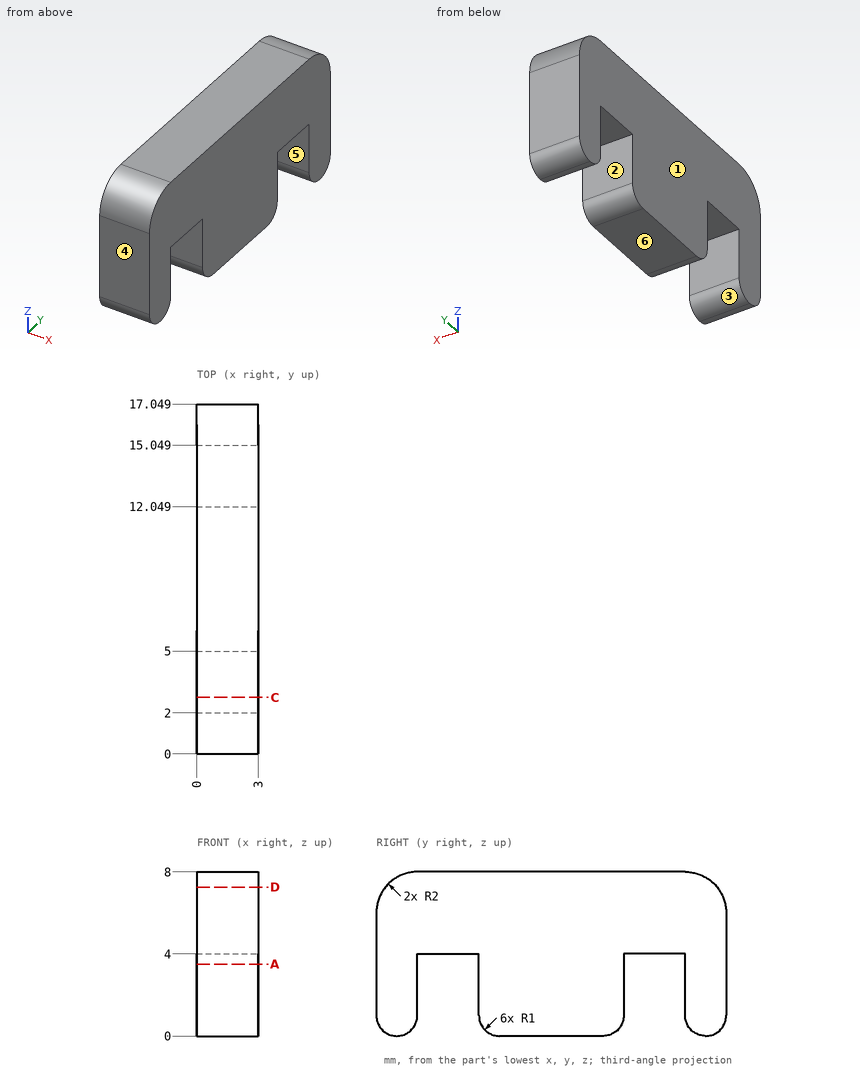
Verification items for this drawing (mm, ordinates from the low corner). A direction names the side the tool comes from. Give positions to 0.01 mm unless a question says otherwise; leave off trailing zeros. Loops run counter-clockwise (first coordinate to the right, second up) from the corner with the lowest first, then second, coordinate; pieces in that order, holes last. Notation, with made-up numbers: M -23,80 L 20,80 A16 ccw 20,95 Z; hole C 76,88 d10. An arc over 180 degrees is marked long. Write item = value, one per line. Start each with the question number.
1. Tool access check on the marked faces 5 and 6. Record the directions out of +Z, -Z, +X, -X, +Y, -Y that give a thin tool (end or side, any length) a straight path to the whole face; none if there is none.
2. Draft check along Y on the marked faces 1, 2, 3 and 4. Enter one of: +Y half, -Y half, draft (parallel to the pull), parting line (faces both ways), or undercut.
3. Section check C-C, the plane y = 2.75. Enter the section's corners in (x, z), plus the area to 3 significant figures.
4. Section check D-D, the plane z = 7.25. Enter the section's corners in (x, y).
5. Thickness scan on probe 1 along Y at (x, z) = (2.25, 1); probe 2 along Z at (x, y) = (1.35, 2.75); probe 3 along Y at (x, z) = (2.65, 6.75) (1 decimal). Record the ranges inside material, lowest first.
6. Section check A-A, the plane z = 3.5. Enter the section's corners in (x, y).
Values follow:
q1.face_5 = -Z, +X, -X
q1.face_6 = -Z, +X, -X, +Y, -Y
q2.face_1 = draft
q2.face_2 = undercut
q2.face_3 = undercut
q2.face_4 = -Y half
q3.outline = M 0,4 L 3,4 L 3,8 L 0,8 Z
q3.area = 12.0 mm^2
q4.outline = M 0,0.44 L 3,0.44 L 3,16.61 L 0,16.61 Z
q5.probe_1 = 0 to 2, 5 to 12.05, 15.05 to 17.05
q5.probe_2 = 4 to 8
q5.probe_3 = 0.1 to 16.9
q6.outline = M 0,0 L 3,0 L 3,2 L 0,2 Z; M 0,5 L 3,5 L 3,12.05 L 0,12.05 Z; M 0,15.05 L 3,15.05 L 3,17.05 L 0,17.05 Z
